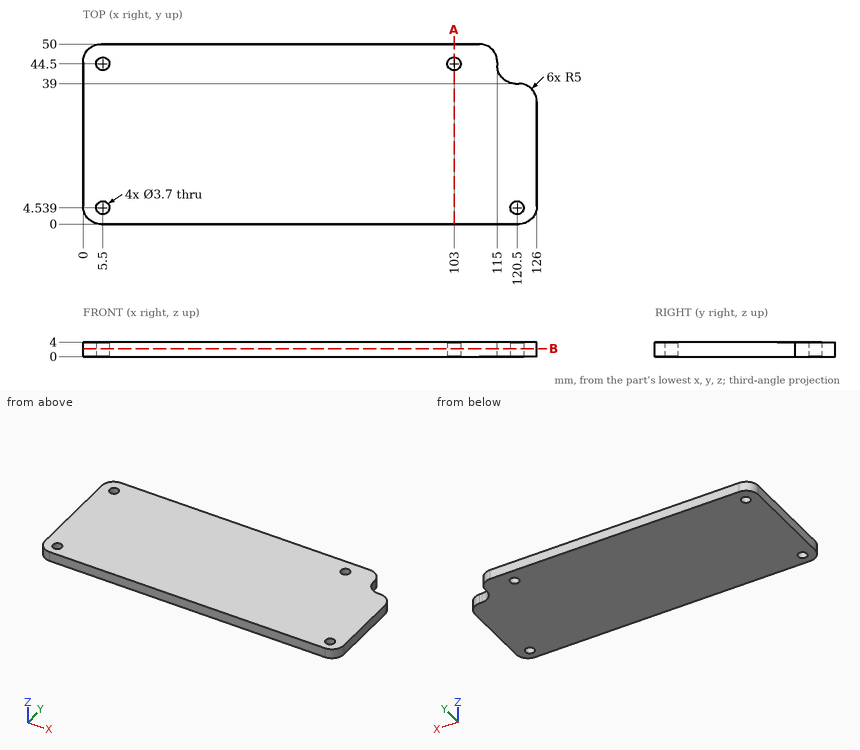
Check sheet for the drawn part. Datum: minimum x, y, z corner. Units: mm. Give positions to 0.01 mm unless a question says otherwise; leave off trailing zeros. Order: outer loops, then holes, each group sorted by start corner. A loop starts at its lowest first (then second) coordinate and runs counter-clockwise, first axis right, second up. Notation, with made-up numbers: (78.5, 23.25) - (106.5, 23.25) arc R17 cw to (106.5, 29.25) - close; hole circle Ø3 at (39.5, 41.5). An arc over 180 degrees is marked (long way). Answer in a Markdown table with one row per item. Add a question column.
Q1. Cross-section at A-A, the plane x = 103. Enter the section's corners in (y, z).
Q2. Cross-section at B-B, the plane z = 2.2. Enter the section's corners in (x, y), then the cut area to 3 significant figures.
Q3. Gauge pin test, flat end, axial feed: pin 1 (3.5 mm diameter, centred on x = 5.5, y = 44.5, fed in from +Z). Record the tip position at first contact, or that the pin passes through.
Q4. Material ranges on probe 1 along Y at (x, z) = (5.5, 1.5); probe 2 along X at (y, z) = (44.5, 2.9); probe 3 along Y at (x, z) = (120.5, 1.6), recorded low to high. Write a range as from..to.
Check values:
| question | item | result |
|---|---|---|
| 1 | outline | (0, 0) - (42.65, 0) - (42.65, 4) - (0, 4) - close; (46.35, 0) - (50, 0) - (50, 4) - (46.35, 4) - close |
| 2 | outline | (0, 5) arc R5 ccw to (5, 0) - (121, 0) arc R5 ccw to (126, 5) - (126, 34) arc R5 ccw to (121, 39) - (120, 39) arc R5 cw to (115, 44) - (115, 45) arc R5 ccw to (110, 50) - (5, 50) arc R5 ccw to (0, 45) - close; hole circle Ø3.7 at (5.5, 4.54); hole circle Ø3.7 at (5.5, 44.5); hole circle Ø3.7 at (103, 44.5); hole circle Ø3.7 at (120.5, 4.54) |
| 2 | area | 6,110 mm^2 |
| 3 | pin 1 | passes through |
| 4 | probe 1 | y = 0..2.69, 6.39..42.65, 46.35..50 |
| 4 | probe 2 | x = 0..3.65, 7.35..101.15, 104.85..115 |
| 4 | probe 3 | y = 0..2.69, 6.39..39 |
